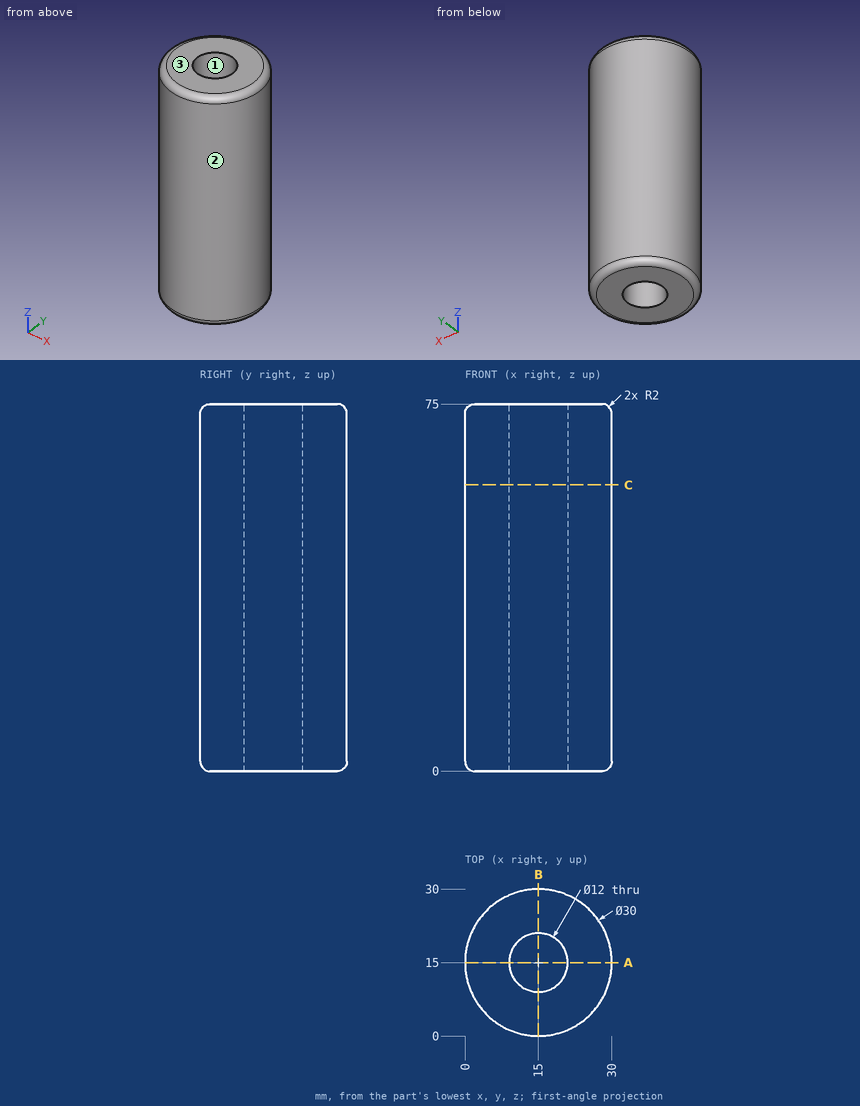
Here's the drawing with two shaded views (mm, measured from the low corner). I have some questions. Coordinates: 2 decimals unless noted, no trailing zeros. Order: outer loops, then holes, each group sorted by start corner. A loop starts at its lowest first (then second) coordinate and runs counter-clockwise, first axis right, second up.
Q1. Suppose I cut it at A-A on y = 15. Please give me the cut outline in (x, z), and give its area (3 significant figures).
Q2. Please list where these lines run through material, in increasing order: L1, parallel to Y at x = 15, z = 46.5; L2, parallel to X at y = 22.5, z = 4; L3, parallel to Y at x = 17.75, z = 58.
Q3. Will these pins go through, and if not, where does the flat tip stop? pin 1 (3 mm diameter, centred on y = 10, z = 35.5, fed in from +X); pin 2 (3 mm diameter, centred on y = 20.5, z = 9.5, fed in from +X); pin 3 (3 mm diameter, centred on x = 13, z = 38, fed in from -Y); pin 4 (10 mm diameter, centred on x = 3.5, y = 6.5, fed in from -Z).
Q4. Suppose I cut it at C-C on z = 58.5. Please give me the cut outline in (x, y).
Q5. Thinking about a two-plate mould opening in Y: for the marked faces 1, 2 and 3, which applies, released by +Y, released by -Y, zero draft, split by the parting line, or undercut?
Answer:
1. outline: (0, 2) arc R2 ccw to (2, 0) - (9, 0) - (9, 75) - (2, 75) arc R2 ccw to (0, 73) - close; (21, 0) - (28, 0) arc R2 ccw to (30, 2) - (30, 73) arc R2 ccw to (28, 75) - (21, 75) - close
1. area: 1,350 mm2
2. L1: y = 0 to 9, 21 to 30
2. L2: x = 2.01 to 27.99
2. L3: y = 0.25 to 9.67, 20.33 to 29.75
3. pin 1: stops at x = 29.59
3. pin 2: stops at x = 29.46
3. pin 3: stops at y = 0.01
3. pin 4: stops at z = 0
4. outline: circle Ø30 at (15, 15); hole circle Ø12 at (15, 15)
5. face 1: undercut
5. face 2: split by the parting line
5. face 3: zero draft
